The listing builds one solid part. Answer for the finished solid, in the listing's coordinates (mm). A direction names the side the tool comes from. Coordinates: 2 decimals unless noted, no trailing zeros. Order: outer loops, then holes, each group sorted by start corner. A loop starts at its lowest first (then second) coordinate and runs counter-clockwise, first axis right, second up. Notation, with made-up numbers: (63.5, -26.5) -> (82.5, -26.5) arc R20 cw to (82.5, 12.5) -> close; hole circle Ø11 at (64.25, -39). An arc over 180 degrees is marked (long way). Answer in a Markdown table with one row per item.
```python
from build123d import *

# Parameters (mm, degrees)
SKETCH1_W               = 35
SKETCH1_H               = 56
BOSS_EXTRUDE1_DEPTH     = 3
SKETCH2_W               = 3
SKETCH2_H               = 26
BOSS_EXTRUDE2_DEPTH     = 30
SKETCH4_R               = 2
CUT_EXTRUDE1_DEPTH      = 33
CUT_EXTRUDE1_DEPTH_BACK = 4
BOSS_EXTRUDE3_DEPTH     = 35
SKETCH6_W               = 29
SKETCH6_H               = 30
CUT_EXTRUDE2_DEPTH      = 30


with BuildPart() as part:
    # Sketch1 → Boss-Extrude1 (new body)
    with BuildSketch(Plane.XY):
        Rectangle(SKETCH1_W, SKETCH1_H)
        with BuildLine():
            Line((-5, 23), (-5, 3))
            ThreePointArc((-5, 3), (-6.5, 1.5), (-8, 3))
            Line((-8, 3), (-8, 23))
            ThreePointArc((-8, 23), (-6.5, 24.5), (-5, 23))
        make_face(mode=Mode.SUBTRACT)
        with BuildLine():
            Line((5, 23), (5, 3))
            ThreePointArc((5, 3), (6.5, 1.5), (8, 3))
            Line((8, 3), (8, 23))
            ThreePointArc((8, 23), (6.5, 24.5), (5, 23))
        make_face(mode=Mode.SUBTRACT)
    extrude(amount=BOSS_EXTRUDE1_DEPTH)

    # Sketch2 → Boss-Extrude2 (add)
    with BuildSketch(Plane.XY.offset(3)):
        with Locations((-16, -15)):
            Rectangle(SKETCH2_W, SKETCH2_H)
        with Locations((16, -15)):
            Rectangle(SKETCH2_W, SKETCH2_H)
    extrude(amount=BOSS_EXTRUDE2_DEPTH)

    # Sketch4 → Cut-Extrude1 (cut, two sides)
    with BuildSketch(Plane.ZY.offset(-14.5)) as cut_extrude1_sk:
        with Locations((18, -15)):
            Circle(SKETCH4_R)
    extrude(amount=CUT_EXTRUDE1_DEPTH, mode=Mode.SUBTRACT)
    extrude(cut_extrude1_sk.sketch, amount=-CUT_EXTRUDE1_DEPTH_BACK, mode=Mode.SUBTRACT)

    # Sketch5 → Boss-Extrude3 (add, through all)
    with BuildSketch(Plane.ZY.offset(17.5)):
        Polygon((3, 28), (33, -2), (3, -2), align=None)
    extrude(amount=-BOSS_EXTRUDE3_DEPTH)

    # Sketch6 → Cut-Extrude2 (cut)
    with BuildSketch(Plane.XY.offset(33)):
        with Locations((0, 13)):
            Rectangle(SKETCH6_W, SKETCH6_H)
    extrude(amount=-CUT_EXTRUDE2_DEPTH, mode=Mode.SUBTRACT)


solid = part.part
```
(1) For a pull along Y with two mould halves and no side action, classify faces 1 (the flat face through (5, 13, 1)), 2 (the flat face through (0, -28, 2)), 3 (the flat face through (0, 28, 1)), 4 (the flat face through (0, 0, 3)) as released by +Y, released by -Y, zero draft, split by the parting line, or undercut.
Check values:
| item | result |
|---|---|
| face 1 | undercut |
| face 2 | released by -Y |
| face 3 | released by +Y |
| face 4 | zero draft |
(2) Which of the six approach directions +Z, -Z, +X, -X, +Y, -Y give full straight-line access (tool end or side, diameter ignored) to faces 5 (the flat face through (14.5, -7, 18)), 6 (the flat face through (-8, 13, 1)), 7 (the cylindrical face through (16, -13, 18))?
Check values:
| item | result |
|---|---|
| face 5 | +Z, +Y, -Y |
| face 6 | +Z, -Z |
| face 7 | +X, -X |
(3) A cutting plane is placed at B-B, the plane z = 6.5. Determine the outline of the cut face in (x, y), then the cut area to 3 significant figures.
Check values:
| item | result |
|---|---|
| outline | (-17.5, -28) -> (-14.5, -28) -> (-14.5, 24.5) -> (-17.5, 24.5) -> close; (14.5, -28) -> (17.5, -28) -> (17.5, 24.5) -> (14.5, 24.5) -> close |
| area | 315 mm² |
(4) A cutting plane is placed at A-A, the plane y = 19.5. Determine the outline of the cut face in (x, z).
Check values:
| item | result |
|---|---|
| outline | (-17.5, 0) -> (-8, 0) -> (-8, 3) -> (-14.5, 3) -> (-14.5, 11.5) -> (-17.5, 11.5) -> close; (-5, 0) -> (5, 0) -> (5, 3) -> (-5, 3) -> close; (8, 0) -> (17.5, 0) -> (17.5, 11.5) -> (14.5, 11.5) -> (14.5, 3) -> (8, 3) -> close |
(5) A cutting plane is placed at D-D, the plane z = 18. Determine the outline of the cut face in (x, y).
Check values:
| item | result |
|---|---|
| outline | (-17.5, -28) -> (-14.5, -28) -> (-14.5, -17) -> (-17.5, -17) -> close; (-17.5, -13) -> (-14.5, -13) -> (-14.5, 13) -> (-17.5, 13) -> close; (14.5, -28) -> (17.5, -28) -> (17.5, -17) -> (14.5, -17) -> close; (14.5, -13) -> (17.5, -13) -> (17.5, 13) -> (14.5, 13) -> close |
(6) Find the intervals of material crossed by line 1 along X through (y, z) = (-8.5, 14.5); line 2 along Z through (x, y) = (-16.65, -15); line 3 along Z through (x, y) = (12, -18.5), in increasing order. Write a range as from..to.
Check values:
| item | result |
|---|---|
| line 1 | -17.5..-14.5, 14.5..17.5 |
| line 2 | 0..16, 20..33 |
| line 3 | 0..3 |
(7) A flat-ended cylindrical pin translates along its axis: pin 1 (5 mm diameter, centred on x = -1.5, y = -21, fed in from +Z). Find the tip coordinate at first contact, or state that the pin passes through.
Check values:
| item | result |
|---|---|
| pin 1 | z = 3 |
(8) A cutting plane is placed at C-C, the plane x = 6.5. Determine the outline of the cut face in (y, z), then the cut area to 3 significant figures.
Check values:
| item | result |
|---|---|
| outline | (-28, 0) -> (1.5, 0) -> (1.5, 3) -> (-28, 3) -> close; (24.5, 0) -> (28, 0) -> (28, 3) -> (24.5, 3) -> close |
| area | 99.0 mm² |
